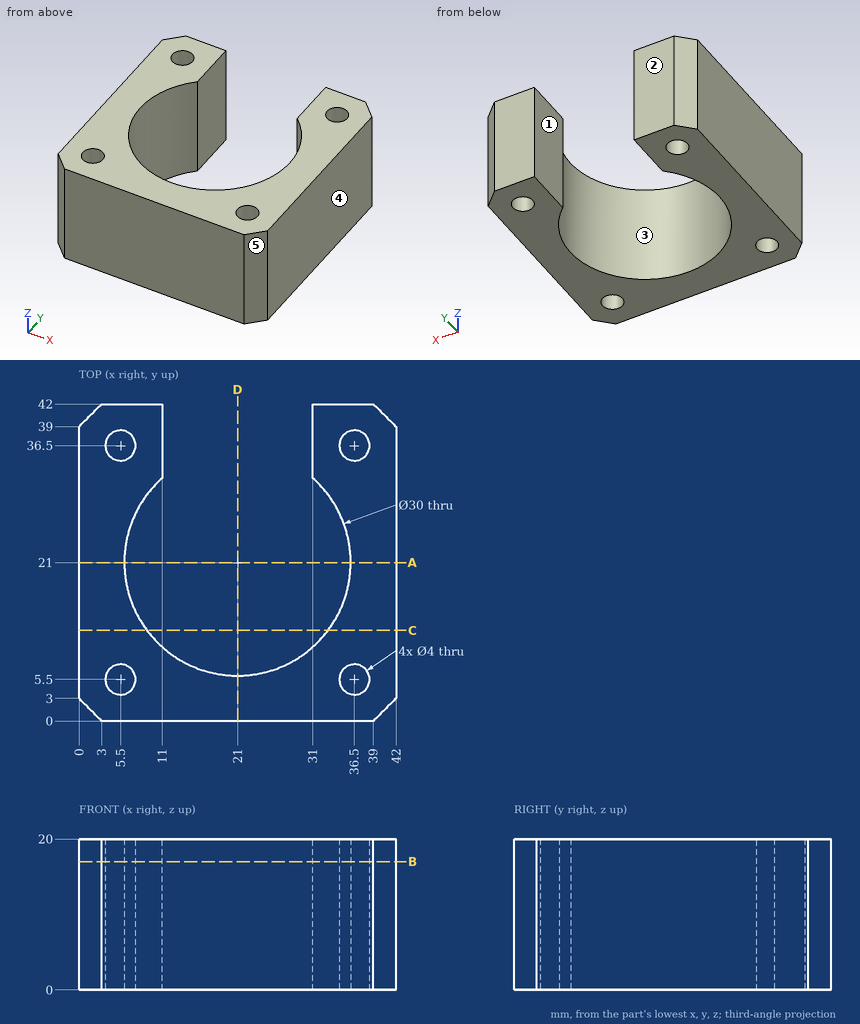
The drawing under review shows one solid part. Ordinate dimensions are in mm from its lowest x, y, z. A direction names the side the tool comes from. Round coordinates to 2 decimals unless told otherwise and drop trailing zeros. Write each loop counter-clockwise with the first axis right and the second up, starting at its lowest first coordinate (ties: lowest second). Pieces come first, ordered by that corner, then holes. Notation, with made-up numbers: (73, 8.5) -> (98, 8.5) arc R24 ccw to (98, 44.5) -> close; hole circle Ø1 at (5, 69.25). An arc over 180 degrees is marked (long way). One line per question, with ' | ' between items. Start each with the question number.
(1) Add section B-B, the plane z = 17. Write out the cut boundary in (x, y), plus the area to 3 significant figures.
(2) For line 1 along Y through (x, z) = (36.5, 6.5); line 2 along X through (y, z) = (20.5, 4.5); line 3 along X through (y, z) = (33.5, 12.25), list the stretches that pass through material, from the lowest coordinate up. Write a range as from..to.
(3) Tool access review of the marked faces 1 and 2: name each direction out of +Z, -Z, +X, -X, +Y, -Y from which nothing blocks a thin tool from reaching the whole face with its end or side.
(4) Add section D-D, the plane x = 21. Write out the cut boundary in (y, z), plus the area to 3 significant figures.
(5) Add section A-A, the plane y = 21. Write out the cut boundary in (x, z).
(6) Insertion check: P1, Ø1.5, axis at x = 15.5, z = 7, coming from the +Y side. The pin has a flat end and moves straight along its axis. Give the tip position at first contact, or say it passes through.
(7) Mouldability with a two-part tool opening along Y and no side actions: class the marked faces 3, 4 and 5 as released by +Y, released by -Y, zero draft, split by the parting line, or undercut.
(8) Add section C-C, the plane y = 12. Write out the cut boundary in (x, z), plus the area to 3 significant figures.
Answer list:
1) outline: (0, 3) -> (3, 0) -> (39, 0) -> (42, 3) -> (42, 39) -> (39, 42) -> (31, 42) -> (31, 32.18) arc R15 cw (long way) to (11, 32.18) -> (11, 42) -> (3, 42) -> (0, 39) -> close; hole circle Ø4 at (5.5, 5.5); hole circle Ø4 at (5.5, 36.5); hole circle Ø4 at (36.5, 5.5); hole circle Ø4 at (36.5, 36.5) | area: 845 mm²
2) line 1: 0..3.5, 7.5..34.5, 38.5..42 | line 2: 0..6.01, 35.99..42 | line 3: 0..11, 31..42
3) face 1: +Z, -Z, +Y | face 2: +Z, -Z, +X, -X, +Y
4) outline: (0, 0) -> (6, 0) -> (6, 20) -> (0, 20) -> close | area: 120 mm²
5) outline: (0, 0) -> (6, 0) -> (6, 20) -> (0, 20) -> close; (36, 0) -> (42, 0) -> (42, 20) -> (36, 20) -> close
6) P1: y = 7.36
7) face 3: undercut | face 4: zero draft | face 5: released by -Y
8) outline: (0, 0) -> (9, 0) -> (9, 20) -> (0, 20) -> close; (33, 0) -> (42, 0) -> (42, 20) -> (33, 20) -> close | area: 360 mm²
